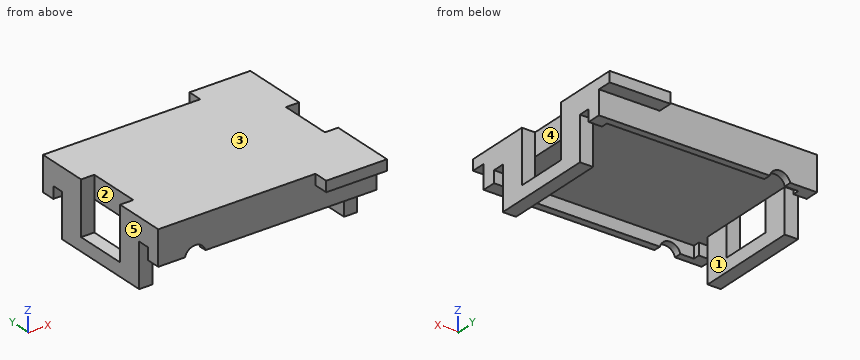
```python
from build123d import *

# Parameters (mm, degrees)
CYLINDER007_R     = 0.8
CYLINDER007_DEPTH = 20
BOX035_W          = 16.5
BOX035_H          = 0.9
BOX035_DEPTH      = 0.9
BOX029_W          = 16.5
BOX029_H          = 0.9
BOX029_DEPTH      = 0.9
BOX032_W          = 16.5
BOX032_H          = 2
BOX032_DEPTH      = 2.4
BOX026_W          = 16.5
BOX026_H          = 2
BOX026_DEPTH      = 2.4
BOX036_W          = 14.5
BOX036_H          = 10.7
BOX036_DEPTH      = 3.3
BOX027_W          = 11.9
BOX027_H          = 1.1
BOX027_DEPTH      = 5
BOX033_W          = 11.9
BOX033_H          = 1.1
BOX033_DEPTH      = 5
BOX028_W          = 4.6
BOX028_H          = 1.1
BOX028_DEPTH      = 4.2
BOX034_W          = 4.6
BOX034_H          = 1.1
BOX034_DEPTH      = 4.2
BOX031_W          = 1
BOX031_H          = 4
BOX031_DEPTH      = 4
BOX030_W          = 1
BOX030_H          = 4
BOX030_DEPTH      = 4
BOX025_W          = 16.5
BOX025_H          = 14
BOX025_DEPTH      = 5


with BuildPart() as cylinder007:
    # Cylinder007 → Cylinder007 (new body)
    with BuildSketch(Plane(origin=(2.8, 10, 2.2), x_dir=(1, 0, 0), z_dir=(0, -1, 0))):
        Circle(CYLINDER007_R)
    extrude(amount=CYLINDER007_DEPTH)


with BuildPart() as cube032:
    # Box035 → Box035 (new body)
    with BuildSketch(Plane(origin=(0, 3.95, 2.4), x_dir=(1, 0, 0), z_dir=(0, 0, 1))):
        with Locations((8.25, 0.45)):
            Rectangle(BOX035_W, BOX035_H)
    extrude(amount=BOX035_DEPTH)


with BuildPart() as compound004:
    # Box029 → Box029 (new body)
    with BuildSketch(Plane(origin=(0, -4.85, 2.4), x_dir=(1, 0, 0), z_dir=(0, 0, 1))):
        with Locations((8.25, 0.45)):
            Rectangle(BOX029_W, BOX029_H)
    extrude(amount=BOX029_DEPTH)

    # Compound004: union Cube032
    add(cube032.part)


with BuildPart() as cube029:
    # Box032 → Box032 (new body)
    with BuildSketch(Plane(origin=(0, -5.95, 0), x_dir=(1, 0, 0), z_dir=(0, 0, 1))):
        with Locations((8.25, 1)):
            Rectangle(BOX032_W, BOX032_H)
    extrude(amount=BOX032_DEPTH)


with BuildPart() as compound005:
    # Box026 → Box026 (new body)
    with BuildSketch(Plane(origin=(0, 3.95, 0), x_dir=(1, 0, 0), z_dir=(0, 0, 1))):
        with Locations((8.25, 1)):
            Rectangle(BOX026_W, BOX026_H)
    extrude(amount=BOX026_DEPTH)

    # Compound005: union Cube029
    add(cube029.part)


with BuildPart() as cube033:
    # Box036 → Box036 (new body)
    with BuildSketch(Plane(origin=(1, -5.35, 0), x_dir=(1, 0, 0), z_dir=(0, 0, 1))):
        with Locations((7.25, 5.35)):
            Rectangle(BOX036_W, BOX036_H)
    extrude(amount=BOX036_DEPTH)


with BuildPart() as cube024:
    # Box027 → Box027 (new body)
    with BuildSketch(Plane(origin=(0, 5.9, 0), x_dir=(1, 0, 0), z_dir=(0, 0, 1))):
        with Locations((5.95, 0.55)):
            Rectangle(BOX027_W, BOX027_H)
    extrude(amount=BOX027_DEPTH)


with BuildPart() as cube030:
    # Box033 → Box033 (new body)
    with BuildSketch(Plane(origin=(0, -7, 0), x_dir=(1, 0, 0), z_dir=(0, 0, 1))):
        with Locations((5.95, 0.55)):
            Rectangle(BOX033_W, BOX033_H)
    extrude(amount=BOX033_DEPTH)


with BuildPart() as cube025:
    # Box028 → Box028 (new body)
    with BuildSketch(Plane(origin=(11.9, -7, 0), x_dir=(1, 0, 0), z_dir=(0, 0, 1))):
        with Locations((2.3, 0.55)):
            Rectangle(BOX028_W, BOX028_H)
    extrude(amount=BOX028_DEPTH)


with BuildPart() as cube031:
    # Box034 → Box034 (new body)
    with BuildSketch(Plane(origin=(11.9, 5.9, 0), x_dir=(1, 0, 0), z_dir=(0, 0, 1))):
        with Locations((2.3, 0.55)):
            Rectangle(BOX034_W, BOX034_H)
    extrude(amount=BOX034_DEPTH)


with BuildPart() as cube028:
    # Box031 → Box031 (new body)
    with BuildSketch(Plane(origin=(0, -2, 1), x_dir=(1, 0, 0), z_dir=(0, 0, 1))):
        with Locations((0.5, 2)):
            Rectangle(BOX031_W, BOX031_H)
    extrude(amount=BOX031_DEPTH)


with BuildPart() as compound003:
    # Box030 → Box030 (new body)
    with BuildSketch(Plane(origin=(15.5, -2, 1), x_dir=(1, 0, 0), z_dir=(0, 0, 1))):
        with Locations((0.5, 2)):
            Rectangle(BOX030_W, BOX030_H)
    extrude(amount=BOX030_DEPTH)

    # Compound003: union Cube028
    add(cube028.part)


with BuildPart() as topcut:
    # Box025 → Box025 (new body)
    with BuildSketch(Plane(origin=(0, -7, 0), x_dir=(1, 0, 0), z_dir=(0, 0, 1))):
        with Locations((8.25, 7)):
            Rectangle(BOX025_W, BOX025_H)
    extrude(amount=BOX025_DEPTH)

    # Cut014: cut Compound003
    add(compound003.part, mode=Mode.SUBTRACT)

    # Cut012: cut Cube031
    add(cube031.part, mode=Mode.SUBTRACT)

    # Cut016: cut Cube025
    add(cube025.part, mode=Mode.SUBTRACT)

    # Cut013: cut Cube030
    add(cube030.part, mode=Mode.SUBTRACT)

    # Cut015: cut Cube024
    add(cube024.part, mode=Mode.SUBTRACT)

    # Cut017: cut Cube033
    add(cube033.part, mode=Mode.SUBTRACT)

    # Cut018: cut Compound005
    add(compound005.part, mode=Mode.SUBTRACT)

    # Cut011: cut Compound004
    add(compound004.part, mode=Mode.SUBTRACT)

    # Cut010: cut Cylinder007
    add(cylinder007.part, mode=Mode.SUBTRACT)


with BuildPart() as topcut_1:
    # Cut010 placement: moved
    add(topcut.part.moved(Location((-8.25, 0, 2.9))))


solid = topcut_1.part
```
Source: CAD feature listing. Evaluate the final solid. Frame: model axes, mm. Face numbers are marked on the shaded views. A direction names the side the tool comes from. Round coordinates to 2 decimals unless told otherwise and drop trailing zeros. Loops run counter-clockwise (first coordinate to the right, second up) from the corner with the lowest first, then second, coordinate; pieces in that order, holes last.
1. Access query for the marked faces 4 and 5. Directions: +Z, -Z, +X, -X, +Y, -Y. A direction counts if a zero-diameter tool reaches every point of the face in a straight line with its end or side. Return the directions, or none.
2. Mould query, pull axis Y, two halves, no side actions, for the marked faces 1, 2 and 3. Classes: released by +Y, released by -Y, zero draft, split by the parting line, or undercut.
3. Section query B-B on z = 3.5. Output: boundary loops of the cut face in (x, y), and give its area (3 significant figures).
4. Section query A-A on y = -1.25. Output: boundary loops of the cut face in (x, z).
5. Section query D-D on z = 5.1. Output: boundary loops of the cut face in (x, y).
6. Section query C-C on x = -3.5. Output: boundary loops of the cut face in (y, z).
7. Ray query, L1, parallel to X at y = 3.5, z = 5; L2, parallel to Y at x = 2.25, z = 5.35; L3, parallel to Y at x = -6.75, z = 7.4. Return the intervals inside material, ascending.
8. Contact query for flat-ended pins moving along their axis: pin 1 (0.6 mm diameter, centred on y = -6, z = 7.5, fed in from -X); pin 2 (3 mm diameter, centred on x = -1.5, y = 1.5, fed in from -Z); pin 3 (1.5 mm diameter, centred on x = -1, z = 6, fed in from -Y); pin 4 (0.5 mm diameter, centred on x = -8, y = 0.5, fed in from +Z). Output: stop coordinate, or through.
Answers below:
1. face 4: +Z, +X
1. face 5: +Z, -Z, -X, +Y, -Y
2. face 1: undercut
2. face 2: undercut
2. face 3: zero draft
3. outline: (-8.25, -3.95) - (-7.25, -3.95) - (-7.25, 3.95) - (-8.25, 3.95) - close; (7.25, -3.95) - (8.25, -3.95) - (8.25, 3.95) - (7.25, 3.95) - close
3. area: 15.8 mm2
4. outline: (-8.25, 2.9) - (-7.25, 2.9) - (-7.25, 3.9) - (-8.25, 3.9) - close; (-7.25, 6.2) - (7.25, 6.2) - (7.25, 7.9) - (-7.25, 7.9) - close; (7.25, 2.9) - (8.25, 2.9) - (8.25, 3.9) - (7.25, 3.9) - close
5. outline: (-8.25, -3.95) - (-7.25, -3.95) - (-7.25, -2) - (-8.25, -2) - close; (-8.25, 2) - (-7.25, 2) - (-7.25, 3.95) - (-8.25, 3.95) - close; (7.25, -3.95) - (8.25, -3.95) - (8.25, -2) - (7.25, -2) - close; (7.25, 2) - (8.25, 2) - (8.25, 3.95) - (7.25, 3.95) - close
6. outline: (-5.9, 5.3) - (-5.35, 5.3) - (-5.35, 6.2) - (5.35, 6.2) - (5.35, 5.3) - (5.9, 5.3) - (5.9, 7.9) - (-5.9, 7.9) - close
7. L1: x = -8.25 to -7.25, 7.25 to 8.25
7. L2: y = -5.9 to -5.35, 5.35 to 5.9
7. L3: y = -5.9 to 5.9
8. pin 1: stops at x = -8.25
8. pin 2: stops at z = 6.2
8. pin 3: stops at y = -5.9
8. pin 4: stops at z = 3.9
